```python
from build123d import *

# Parameters (mm, degrees)
F0_W      = 130
F0_H      = 130
F1_DEPTH  = 60
F2_W      = 110
F2_H      = 110
F3_DEPTH  = 50
F4_W      = 89
F4_H      = 40
F5_DEPTH  = 4
F6_R      = 7
F7_W      = 10
F7_H      = 4
F8_DEPTH  = 4
F9_W      = 10
F9_H      = 4
F10_DEPTH = 4
F11_W     = 10
F11_H     = 10
F12_DEPTH = 4


with BuildPart() as f1:
    # F0 (on Top) → F1 (new body)
    with BuildSketch(Plane.XY):
        Rectangle(F0_W, F0_H)
    extrude(amount=F1_DEPTH)

    # F2 (on Top) → F3 (cut)
    with BuildSketch(Plane.XY):
        Rectangle(F2_W, F2_H)
    extrude(amount=F3_DEPTH, mode=Mode.SUBTRACT)

    # F4 (on face) → F5 (cut)
    with BuildSketch(Plane.XY.offset(60)):
        with Locations((20.5, 0)):
            Rectangle(F4_W, F4_H)
    extrude(amount=-F5_DEPTH, mode=Mode.SUBTRACT)

    # F6
    f6_edges = [f1.edges().sort_by_distance(p)[0] for p in [
        (55, -55, 25),
        (55, 55, 25),
        (-55, 55, 25),
        (-55, -55, 25),
    ]]
    fillet(f6_edges, radius=F6_R)

    # F7 (on face) → F8 (cut)
    with BuildSketch(Plane.XY):
        with Locations((-60, -39.780788)):
            Rectangle(F7_W, F7_H)
    extrude(amount=F8_DEPTH, mode=Mode.SUBTRACT)

    # F9 (on face) → F10 (cut)
    with BuildSketch(Plane.XY):
        with Locations((-60, -47.136784)):
            Rectangle(F9_W, F9_H)
    extrude(amount=F10_DEPTH, mode=Mode.SUBTRACT)

    # F11 (on face) → F12 (cut)
    with BuildSketch(Plane.XY):
        with Locations((-60, 45)):
            Rectangle(F11_W, F11_H)
    extrude(amount=F12_DEPTH, mode=Mode.SUBTRACT)


solid = f1.part
```
Input: part model. Units: mm. Frame: model coordinates. A direction names the side the tool comes from. Coordinates: 2 decimals unless noted, no trailing zeros. Write each loop counter-clockwise with the first axis right and the second up, starting at its lowest first coordinate (ties: lowest second). Pieces come first, ordered by that corner, then holes. Notation, with made-up numbers: M -7.5,43 L 15.5,43 A31 ccw 15.5,73 Z; hole C -33,85.5 d1. An arc over 180 degrees is marked long. Use one line per item in the form item = value.
Q1. Section B-B (z = 22). Return loops of the section in (x, y), plus the area to 3 significant figures.
Answer below:
outline = M -65,-65 L 65,-65 L 65,65 L -65,65 Z; hole M -55,-48 A7 ccw -48,-55 L 48,-55 A7 ccw 55,-48 L 55,48 A7 ccw 48,55 L -48,55 A7 ccw -55,48 Z
area = 4,840 mm²
Q2. Set-up query: faces 5 (the face through (20, 0, 56)), 6 (the face through (-1, 1, 50)), 7 (the face through (-60, -40, 4)). Return all of +Z, -Z, +X, -X, +Y, -Y with unobstructed straight access to the full face (end or side cutting, diameter ignored); none if empty.
Answer below:
face_5 = +Z, +X
face_6 = -Z
face_7 = -Z, -X
Q3. Draft query along Y for faces 1 (the face through (-60, -41.781, 2)), 2 (the face through (52.9, -53, 25.4)), 3 (the face through (-1, 65, 30)), 4 (the face through (65, -1, 30)). Return one class per face: released by +Y, released by -Y, zero draft, split by the parting line, or undercut.
Answer below:
face_1 = undercut
face_2 = undercut
face_3 = released by +Y
face_4 = zero draft
Q4. Section A-A (y = 43.5). Return loops of the section in (x, z), plus the area to 3 significant figures.
Answer below:
outline = M -65,4 L -55,4 L -55,50 L 55,50 L 55,0 L 65,0 L 65,60 L -65,60 Z
area = 2,260 mm²
Q5. Section D-D (y = -17). Return loops of the section in (x, z).
Answer below:
outline = M -65,0 L -55,0 L -55,50 L 55,50 L 55,0 L 65,0 L 65,56 L -24,56 L -24,60 L -65,60 Z
Q6. Section C-C (x = 6.5). Return loops of the section in (y, z).
Answer below:
outline = M -65,0 L -55,0 L -55,50 L 55,50 L 55,0 L 65,0 L 65,60 L 20,60 L 20,56 L -20,56 L -20,60 L -65,60 Z
Q7. Material intervals for probe 1 along Y at (x, z) = (-18, 7); probe 2 along Z at (x, y) = (-9.5, 42), sorted ascending. Write a range as from..to.
Answer below:
probe_1 = -65..-55, 55..65
probe_2 = 50..60
Q8. First-contact query: pin 1 (1.2 mm diameter, centred on x = -62, y = -46.5, fed in from -Z); pin 2 (0.6 mm diameter, centred on y = 49, z = 1.5, fed in from -X). Flat tips, straight axial feed; report the tip coordinate or a pass-through.
Answer below:
pin_1 = 4
pin_2 = -55
